from build123d import *

# Parameters (mm, degrees)
SKETCH1_W           = 80
SKETCH1_H           = 80
BOSS_EXTRUDE2_DEPTH = 1.5
SKETCH2_R           = 31.5
SKETCH2_R_2         = 30
CUT_EXTRUDE2_DEPTH  = 0.75


with BuildPart() as part:
    # Sketch1 → Boss-Extrude2 (new body)
    with BuildSketch(Plane(origin=(0, 0, 0), x_dir=(1, 0, 0), z_dir=(0, 1, 0))):
        with Locations((-0.604095773, 0)):
            Rectangle(SKETCH1_W, SKETCH1_H)
    extrude(amount=BOSS_EXTRUDE2_DEPTH)

    # Sketch2 → Cut-Extrude2 (cut)
    with BuildSketch(Plane(origin=(0, 1.5, 0), x_dir=(1, 0, 0), z_dir=(0, 1, 0))):
        with Locations(Location((0, 0, 0), (0, 0, 270))):
            Circle(SKETCH2_R)
        with Locations(Location((0, 0, 0), (0, 0, 270))):
            Circle(SKETCH2_R_2, mode=Mode.SUBTRACT)
    extrude(amount=-CUT_EXTRUDE2_DEPTH, mode=Mode.SUBTRACT)


solid = part.part
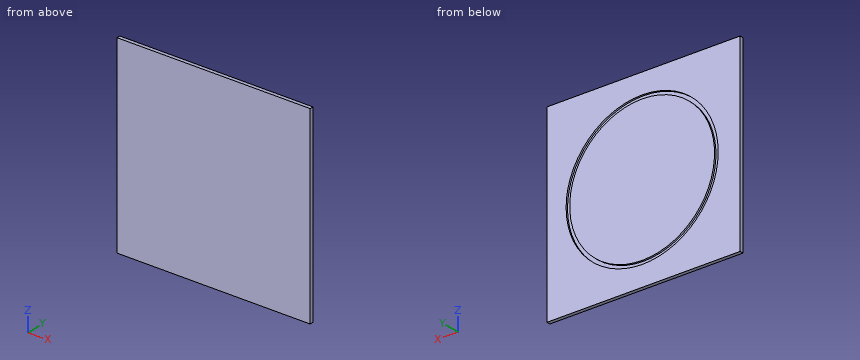
Could you check a few things on this model? Use its own coordinates, in mm. Give positions to 0.01 mm unless a question says otherwise; leave off trailing zeros. Order: outer loops, then holes, each group sorted by start corner. A loop starts at its lowest first (then second) coordinate and runs counter-clockwise, first axis right, second up. Notation, with made-up numbers: (43.5, -39) - (64.5, -39) arc R21 cw to (64.5, -24) - close; hole circle Ø3 at (-29, 74.5). An arc over 180 degrees is marked (long way). Return JSON: item names as keys, results as strings. Group by question number.
Q1. Suppose I cut it at C-C, the plane x = 0. Please give me the cut outline in (y, z), and give its area (3 significant figures).
Q2. Please list where these lines run through material, in increasing order: line 1 along X through (y, z) = (1.05, 0); line 2 along Z through (x, y) = (9, 1); line 3 along X through (y, z) = (0.8, 18). Write a range as [from, to].
Q3. Suppose I cut it at A-A, the plane y = 1. Please give me the cut outline in (x, z).
Q4. Suppose I cut it at B-B, the plane z = 0. Please give me the cut outline in (x, y), and give its area (3 significant figures).
Resolved:
{
 "1": {"outline": "(0, -40) - (1.5, -40) - (1.5, -31.5) - (0.75, -31.5) - (0.75, -30) - (1.5, -30) - (1.5, 30) - (0.75, 30) - (0.75, 31.5) - (1.5, 31.5) - (1.5, 40) - (0, 40) - close", "area": "118 mm2"},
 "2": {"line 1": "x = [-40.6, -31.5], [-30, 30], [31.5, 39.4]", "line 2": "z = [-40, -30.19], [-28.62, 28.62], [30.19, 40]", "line 3": "x = [-40.6, -25.85], [-24, 24], [25.85, 39.4]"},
 "3": {"outline": "(-40.6, -40) - (39.4, -40) - (39.4, 40) - (-40.6, 40) - close; circle Ø60 at (0, 0); hole circle Ø63 at (0, 0)"},
 "4": {"outline": "(-40.6, 0) - (39.4, 0) - (39.4, 1.5) - (31.5, 1.5) - (31.5, 0.75) - (30, 0.75) - (30, 1.5) - (-30, 1.5) - (-30, 0.75) - (-31.5, 0.75) - (-31.5, 1.5) - (-40.6, 1.5) - close", "area": "118 mm2"}
}
